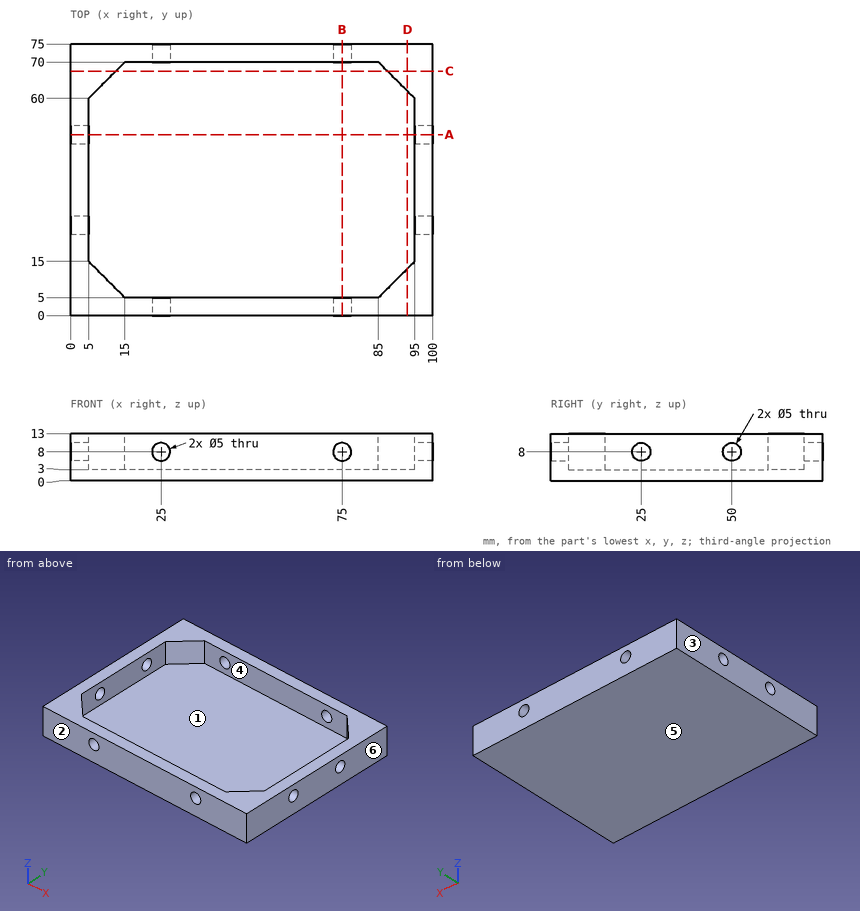
Geometry: see drawing. Coordinates: mm, zero at the bounding-box minimum. A direction names the side the tool comes from. Round coordinates to 2 decimals unless told otherwise and drop trailing zeros. Loops run counter-clockwise (first coordinate to the right, second up) from the corner with the lowest first, then second, coordinate; pieces in that order, holes last. Notation, with made-up numbers: (-37, 35) - (-30, 35) arc R20 ccw to (-30, 58) - close; hole circle Ø4 at (46.25, 73). An arc over 180 degrees is marked (long way). One line per item, written item: value. Start each with the question number.
(1) Section A-A, the plane y = 50. Return loops of the section in (x, z).
(2) Ray query, line 1 (X direction, y = 73.3, z = 8); line 2 (X direction, y = 16, z = 4.5); line 3 (Z direction, x = 1.4, y = 25). Return the intervals inside material, ascending. Write a range as [from, to].
(3) Section D-D, the plane x = 93. Return loops of the section in (y, z).
(4) Section B-B, the plane x = 75. Return loops of the section in (y, z).
(5) Draft query along X for the marked faces 3, 4, 5 and 6. Return one class per face: +X half, -X half, draft (parallel to the pull), parting line (faces both ways), or undercut.
(6) Contact query for a flat-ended pin moving along its axis: P1, Ø12, axis at x = 52, y = 23, coming from the +Z side. Output: stop coordinate, or through.
(7) Access query for the marked faces 1 and 2. Directions: +Z, -Z, +X, -X, +Y, -Y. A direction counts if a zero-diameter tool reaches every point of the face in a straight line with its end or side. Return the directions, or none.
(8) Section C-C, the plane y = 67.5. Return loops of the section in (x, z).
Results below:
1. outline: (0, 0) - (100, 0) - (100, 5.5) - (95, 5.5) - (95, 3) - (5, 3) - (5, 5.5) - (0, 5.5) - close; (0, 10.5) - (5, 10.5) - (5, 13) - (0, 13) - close; (95, 10.5) - (100, 10.5) - (100, 13) - (95, 13) - close
2. line 1: [0, 22.5], [27.5, 72.5], [77.5, 100]
2. line 2: [0, 5], [95, 100]
2. line 3: [0, 5.5], [10.5, 13]
3. outline: (0, 0) - (75, 0) - (75, 13) - (62, 13) - (62, 3) - (13, 3) - (13, 13) - (0, 13) - close
4. outline: (0, 0) - (75, 0) - (75, 5.5) - (70, 5.5) - (70, 3) - (5, 3) - (5, 5.5) - (0, 5.5) - close; (0, 10.5) - (5, 10.5) - (5, 13) - (0, 13) - close; (70, 10.5) - (75, 10.5) - (75, 13) - (70, 13) - close
5. face 3: -X half
5. face 4: undercut
5. face 5: draft
5. face 6: +X half
6. P1: z = 3
7. face 1: +Z
7. face 2: +Z, -Z, +X, -X, -Y
8. outline: (0, 0) - (100, 0) - (100, 13) - (87.5, 13) - (87.5, 3) - (12.5, 3) - (12.5, 13) - (0, 13) - close
